```python
from build123d import *

# Parameters (mm, degrees)
SKETCH1_W           = 139.7
SKETCH1_H           = 139.7
BOSS_EXTRUDE1_DEPTH = 6.35
SKETCH2_R           = 3.175
CUT_EXTRUDE1_DEPTH  = 6.35
SKETCH4_R           = 3.175
SKETCH4_R_2         = 1.42875
BOSS_EXTRUDE2_DEPTH = 7.9375


with BuildPart() as part:
    # Sketch1 → Boss-Extrude1 (new body)
    with BuildSketch(Plane(origin=(0, 0, 0), x_dir=(1, 0, 0), z_dir=(0, 1, 0))):
        Rectangle(SKETCH1_W, SKETCH1_H)
    extrude(amount=BOSS_EXTRUDE1_DEPTH)

    # Sketch2 → Cut-Extrude1 (cut)
    with BuildSketch(Plane(origin=(0, 6.35, 0), x_dir=(1, 0, 0), z_dir=(0, 1, 0))):
        with Locations(Location((-63.5, -63.5, 0), (0, 0, 270))):
            Circle(SKETCH2_R)
        with Locations(Location((63.5, -63.5, 0), (0, 0, 90))):
            Circle(SKETCH2_R)
        with Locations(Location((63.5, 63.5, 0), (0, 0, 270))):
            Circle(SKETCH2_R)
        with Locations(Location((-63.5, 63.5, 0), (0, 0, 90))):
            Circle(SKETCH2_R)
    extrude(amount=-CUT_EXTRUDE1_DEPTH, mode=Mode.SUBTRACT)

    # Sketch4 → Boss-Extrude2 (add)
    # profile 1 of 4: a face of its own
    with BuildSketch(Plane(origin=(0, 6.35, 0), x_dir=(1, 0, 0), z_dir=(0, 1, 0))):
        with Locations(Location((-57.15, 26.9875, 0), (0, 0, 270))):
            Circle(SKETCH4_R)
        with Locations(Location((-57.15, 26.9875, 0), (0, 0, 270))):
            Circle(SKETCH4_R_2, mode=Mode.SUBTRACT)
    # profile 2 of 4: a face of its own
    with BuildSketch(Plane(origin=(0, 6.35, 0), x_dir=(1, 0, 0), z_dir=(0, 1, 0))):
        with Locations(Location((-57.15, -26.9875, 0), (0, 0, 270))):
            Circle(SKETCH4_R)
        with Locations(Location((-57.15, -26.9875, 0), (0, 0, 270))):
            Circle(SKETCH4_R_2, mode=Mode.SUBTRACT)
    # profile 3 of 4: a face of its own
    with BuildSketch(Plane(origin=(0, 6.35, 0), x_dir=(1, 0, 0), z_dir=(0, 1, 0))):
        with Locations(Location((57.15, -26.9875, 0), (0, 0, 270))):
            Circle(SKETCH4_R)
        with Locations(Location((57.15, -26.9875, 0), (0, 0, 270))):
            Circle(SKETCH4_R_2, mode=Mode.SUBTRACT)
    # profile 4 of 4: a face of its own
    with BuildSketch(Plane(origin=(0, 6.35, 0), x_dir=(1, 0, 0), z_dir=(0, 1, 0))):
        with Locations(Location((57.15, 26.9875, 0), (0, 0, 270))):
            Circle(SKETCH4_R)
        with Locations(Location((57.15, 26.9875, 0), (0, 0, 270))):
            Circle(SKETCH4_R_2, mode=Mode.SUBTRACT)
    extrude(amount=BOSS_EXTRUDE2_DEPTH)


solid = part.part
```
Design review of the part built by this model. Coordinates are the model's own, in mm. A direction names the side the tool comes from. Coordinates: 2 decimals unless noted, no trailing zeros. Order: outer loops, then holes, each group sorted by start corner. A loop starts at its lowest first (then second) coordinate and runs counter-clockwise, first axis right, second up. Notation, with made-up numbers: (15, 83) -> (30, 83) arc R28 cw to (30, 107) -> close; hole circle Ø7 at (-2, -15.5). An arc over 180 degrees is marked (long way). One line per item, written item: value. Start each with the question number.
Q1. Insertion check: pin 1 Ø2.5 at (x, z) = (57.15, -26.99) entering from +Y; pin 2 Ø5 at (x, z) = (-63.5, 63.5) entering from +Y. Each pin has a flat end and moves straight along its axis. Give the tip position at first contact, or say it passes through.
Q2. Take a section at A-A, the plane y = 8.75. Give the number of separate pieces and of enclosed holes in the cut face, then the cut area to 3 significant figures.
Q3. Take a section at D-D, the plane x = 25. State the section outline as (y, z) points, then the cut area to 3 significant figures.
Q4. Mouldability with a two-part tool opening along X and no side actions: class faces 1 (the cylindrical face through (54.05, 10.26, -27.68)), 2 (the flat face through (69.85, 3, 1)), 3 (the flat face through (-69.85, 3, 1)), 4 (the flat face through (-1, 3, 69.85)) as pulls with the +X half, pulls with the -X half, needs draft (parallel to the pull), parting line crosses it, or undercut.
Q5. Take a section at B-B, the plane z = -63.5. State the section outline as (x, y) points (3 decimals).
Q6. For probe 1 along X at (y, z) = (3.75, 63.5) (3 decimals); probe 2 along Z at (x, y) = (-58, 13); probe 3 along Y at (x, z) = (-62, 38.5), list the stretches that pass through material, from the lowest coordinate up.
Q7. Take a section at C-C, the plane x = 63.5. State the section outline as (y, z) points (3 decimals).
Q8. Tool access review of faces 5 (the flat face through (-1, 0, -1)), 6 (the cylindrical face through (-55, 10.26, 24.65)): name each direction out of +Z, -Z, +X, -X, +Y, -Y from which nothing blocks a thin tool from reaching the whole face with its end or side.
Values follow:
1. pin 1: stops at y = 6.35
1. pin 2: passes through
2. separate pieces: 4
2. enclosed holes: 4
2. area: 101 mm2
3. outline: (0, -69.85) -> (6.35, -69.85) -> (6.35, 69.85) -> (0, 69.85) -> close
3. area: 887 mm2
4. face 1: undercut
4. face 2: pulls with the +X half
4. face 3: pulls with the -X half
4. face 4: needs draft
5. outline: (-69.85, 0) -> (-66.675, 0) -> (-66.675, 6.35) -> (-69.85, 6.35) -> close; (-60.325, 0) -> (60.325, 0) -> (60.325, 6.35) -> (-60.325, 6.35) -> close; (66.675, 0) -> (69.85, 0) -> (69.85, 6.35) -> (66.675, 6.35) -> close
6. probe 1: x = -69.85 to -66.675, -60.325 to 60.325, 66.675 to 69.85
6. probe 2: z = -30.05 to -28.14, -25.84 to -23.93, 23.93 to 25.84, 28.14 to 30.05
6. probe 3: y = 0 to 6.35
7. outline: (0, -69.85) -> (6.35, -69.85) -> (6.35, -66.675) -> (0, -66.675) -> close; (0, -60.325) -> (6.35, -60.325) -> (6.35, 60.325) -> (0, 60.325) -> close; (0, 66.675) -> (6.35, 66.675) -> (6.35, 69.85) -> (0, 69.85) -> close
8. face 5: +Z, -Z, +X, -X, -Y
8. face 6: +Y
